Verification items for the finished model (mm, model axes). A direction names the side the tool comes from. Give positions to 0.01 mm unless a question says otherwise; leave off trailing zeros. Loops run counter-clockwise (first coordinate to the right, second up) from the corner with the lowest first, then second, coordinate; pieces in that order, holes last. Notation, with made-up numbers: (12.5, 17.25) - (33.5, 17.25) arc R14 cw to (33.5, 36.25) - close; hole circle Ø4 at (70.5, 1.5). An arc over 180 degrees is marked (long way). Use one line per item in the form item = value.
```python
from build123d import *

# Parameters (mm, degrees)
SKETCH1_W           = 203.2
SKETCH1_H           = 203.2
BOSS_EXTRUDE1_DEPTH = 6.35
SKETCH3_R           = 8.334375
SKETCH3_W           = 101.6
SKETCH3_H           = 38.1
CUT_EXTRUDE1_DEPTH  = 144.824345992
SKETCH4_W           = 114.3
SKETCH4_H           = 6.604
CUT_EXTRUDE2_DEPTH  = 144.824345992
SKETCH5_W           = 12.7
SKETCH5_H           = 3.175
CUT_EXTRUDE3_DEPTH  = 144.824345992


with BuildPart() as part:
    # Sketch1 → Boss-Extrude1 (new body)
    with BuildSketch(Plane(origin=(0, 0, 0), x_dir=(1, 0, 0), z_dir=(0, 1, 0))):
        Rectangle(SKETCH1_W, SKETCH1_H)
    extrude(amount=BOSS_EXTRUDE1_DEPTH)

    # Sketch3 → Cut-Extrude1 (cut, through all)
    with BuildSketch(Plane(origin=(0, 6.35, 0), x_dir=(1, 0, 0), z_dir=(0, 1, 0))):
        with Locations(Location((-76.2, 76.2, 0), (0, 0, 270))):
            Circle(SKETCH3_R)
        with Locations(Location((76.2, 76.2, 0), (0, 0, 270))):
            Circle(SKETCH3_R)
        with Locations(Location((-76.2, -76.2, 0), (0, 0, 270))):
            Circle(SKETCH3_R)
        with Locations(Location((76.2, -76.2, 0), (0, 0, 270))):
            Circle(SKETCH3_R)
        with Locations((0, 82.55)):
            Rectangle(SKETCH3_W, SKETCH3_H)
    extrude(amount=-CUT_EXTRUDE1_DEPTH, mode=Mode.SUBTRACT)

    # Sketch4 → Cut-Extrude2 (cut, through all)
    with BuildSketch(Plane(origin=(0, 6.35, 0), x_dir=(1, 0, 0), z_dir=(0, 1, 0))):
        with Locations((0, -50.8)):
            Rectangle(SKETCH4_W, SKETCH4_H)
        with Locations((0, 25.4)):
            Rectangle(SKETCH4_W, SKETCH4_H)
        with Locations((0, -76.2)):
            Rectangle(SKETCH4_W, SKETCH4_H)
        Rectangle(SKETCH4_W, SKETCH4_H)
        with Locations((0, -25.4)):
            Rectangle(SKETCH4_W, SKETCH4_H)
    extrude(amount=-CUT_EXTRUDE2_DEPTH, mode=Mode.SUBTRACT)

    # Sketch5 → Cut-Extrude3 (cut, through all)
    with BuildSketch(Plane(origin=(0, 6.35, 0), x_dir=(1, 0, 0), z_dir=(0, 1, 0))):
        with Locations((-25.4, 46.101)):
            Rectangle(SKETCH5_W, SKETCH5_H)
        with Locations((25.4, 46.101)):
            Rectangle(SKETCH5_W, SKETCH5_H)
        with Locations((-25.4, 14.101)):
            Rectangle(SKETCH5_W, SKETCH5_H)
        with Locations((25.4, 14.101)):
            Rectangle(SKETCH5_W, SKETCH5_H)
        with Locations((-25.4, -36.699)):
            Rectangle(SKETCH5_W, SKETCH5_H)
        with Locations((25.4, -36.699)):
            Rectangle(SKETCH5_W, SKETCH5_H)
    extrude(amount=-CUT_EXTRUDE3_DEPTH, mode=Mode.SUBTRACT)


solid = part.part
```
1. Section check A-A, the plane x = -76.2. Record the cut outline in (y, z), then the cut area to 3 significant figures.
Result set:
outline = (0, -101.6) - (6.35, -101.6) - (6.35, -84.53) - (0, -84.53) - close; (0, -67.87) - (6.35, -67.87) - (6.35, 67.87) - (0, 67.87) - close; (0, 84.53) - (6.35, 84.53) - (6.35, 101.6) - (0, 101.6) - close
area = 1,080 mm²
2. Draft check along Z on faces 3 (the cylindrical face through (-73.7, 3.22, 84.15)), 4 (the flat face through (50.8, 3, -82)). Enter one of: released by +Z, released by -Z, zero draft, split by the parting line, or undercut.
Result set:
face_3 = undercut
face_4 = zero draft
3. Tool access check on faces 1 (the flat face through (-50.8, 3, -82)), 2 (the flat face through (57.15, 3, -25)). Record the directions out of +Z, -Z, +X, -X, +Y, -Y that give a thin tool (end or side, any length) a straight path to the whole face; none if there is none.
Result set:
face_1 = -Z, +Y, -Y
face_2 = +Y, -Y
4. Scan lines: probe 1 along X at (y, z) = (4.5, 76.2); probe 2 along X at (y, z) = (5, -76.2); probe 3 along Z at (x, y) = (-35.5, 5). Record each from-to range of solid material in increasing order.
Result set:
probe_1 = -101.6 to -84.53, -67.87 to -57.15, 57.15 to 67.87, 84.53 to 101.6
probe_2 = -101.6 to -84.53, -67.87 to -50.8, 50.8 to 67.87, 84.53 to 101.6
probe_3 = -63.5 to -28.7, -22.1 to -3.3, 3.3 to 22.1, 28.7 to 47.5, 54.1 to 72.9, 79.5 to 101.6
5. Section check C-C, the plane z = -76.2. Record the cut outline in (x, y), then the cut area to 3 significant figures.
Result set:
outline = (-101.6, 0) - (-84.53, 0) - (-84.53, 6.35) - (-101.6, 6.35) - close; (-67.87, 0) - (-50.8, 0) - (-50.8, 6.35) - (-67.87, 6.35) - close; (50.8, 0) - (67.87, 0) - (67.87, 6.35) - (50.8, 6.35) - close; (84.53, 0) - (101.6, 0) - (101.6, 6.35) - (84.53, 6.35) - close
area = 433 mm²
6. Depth check by flat-ended pin: pin 1 Ø15 at (x, z) = (76.2, -76.2) entering from +Y; pin 2 Ø1.9 at (x, y) = (-8, 3.5) entering from -Z. Enter the tip coordinate at first touch or a pass-through.
Result set:
pin_1 = through
pin_2 = -63.5
7. Section check D-D, the plane x = 4.5. Record the cut outline in (y, z), then the cut area to 3 significant figures.
Result set:
outline = (0, -63.5) - (6.35, -63.5) - (6.35, -28.7) - (0, -28.7) - close; (0, -22.1) - (6.35, -22.1) - (6.35, -3.3) - (0, -3.3) - close; (0, 3.3) - (6.35, 3.3) - (6.35, 22.1) - (0, 22.1) - close; (0, 28.7) - (6.35, 28.7) - (6.35, 47.5) - (0, 47.5) - close; (0, 54.1) - (6.35, 54.1) - (6.35, 72.9) - (0, 72.9) - close; (0, 79.5) - (6.35, 79.5) - (6.35, 101.6) - (0, 101.6) - close
area = 839 mm²
8. Section check B-B, the plane z = 51. Record the cut outline in (x, y), then the cut area to 3 significant figures.
Result set:
outline = (-101.6, 0) - (-57.15, 0) - (-57.15, 6.35) - (-101.6, 6.35) - close; (57.15, 0) - (101.6, 0) - (101.6, 6.35) - (57.15, 6.35) - close
area = 565 mm²
